CAD build for the part. Positions are in the model's coordinates, mm. Face numbers are marked on the shaded views. A direction names the side the tool comes from. Coordinates: 2 decimals unless noted, no trailing zeros. Order: outer loops, then holes, each group sorted by start corner. A loop starts at its lowest first (then second) coordinate and runs counter-clockwise, first axis right, second up. Notation, with made-up numbers: (13.5, -16.5) - (71.5, -16.5) arc R22 cw to (71.5, 10.5) - close; hole circle Ø8 at (-32.5, -33). An arc over 180 degrees is marked (long way). Write each question's results on one line, items separated by ' | '. Start each with the question number.
Q1. Which spindle directions (+Z, -Z, +X, -X, +Y, -Y) get a long thin tool onto all of the face, cutting with end or side? Do the marked faces 1 and 2. Say none if no direction does.
Q2. Wall check: probe 1 along Y at (x, z) = (-4.5, -0.75); probe 2 along X at (y, z) = (16.25, 0.5); probe 3 along X at (y, z) = (14.5, 1). Give the ranges that are in metal, low to high.
Q3. Band-saw the part on A-A, the plane y = 13.5. Write the cut outline in (x, z), then the cut area to 3 significant figures.
Q4. Pin check, flat tips, straight feed: P1, Ø1.5, axis at x = 0.5, y = 8.5, coming from the -Z side; P2, Ø2, axis at x = -3.5, y = 16.5, coming from the -Z side; P3, Ø2, axis at x = 4, z = 2, coming from the -Y side; P4, Ø3, axis at y = 13.5, z = -1, coming from the -X side. Stop position of each tip, or through.
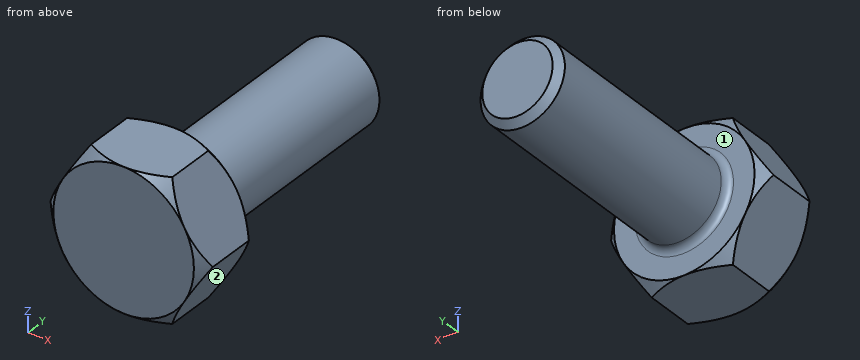
Autodesk Inventor part; units mm, degrees
ref_plane "YZ Plane" through (0, 0, 0) normal (1, 0, 0) x (0, 1, 0)
ref_plane "XZ Plane" through (0, 0, 0) normal (0, 1, 0) x (-1, 0, 0)
ref_plane "XY Plane" through (0, 0, 0) normal (0, 0, 1) x (1, 0, 0)
sketch "Esboço1" plane through (0, 0, 0) normal (0, 1, 0) x (-1, 0, 0)
  circle A0 centre (0, 0) radius 3
  line L0 (-2.8868, -5) -> (-5.7735, 0)
  line L1 (-5.7735, 0) -> (-2.8868, 5)
  line L2 (-2.8868, 5) -> (2.8868, 5)
  line L3 (2.8868, 5) -> (5.7735, 0)
  line L4 (5.7735, 0) -> (2.8868, -5)
  line L5 (2.8868, -5) -> (-2.8868, -5)
  dimension "d0" = 6
extrude "Extrusão1" add sketch "Esboço1" along normal blind 5
sketch "Esboço2" plane through (0, 0, 0) normal (1, 0, 0) x (0, 1, 0)
  point P0 (0, 0)
chamfer "Chanfro1" distance 0.5 angle 45 2 edges at (3, 0, 0) (3, 5, 0)
sketch "Esboço5" plane through (0, 0, 0) normal (0, -1, 0) x (1, 0, 0)
  circle A0 centre (0, 0) radius 5
extrude "Extrusão2" cut sketch "Esboço5" against normal through all draft 45 keep common part
sketch "Esboço6" plane through (0, 5, 0) normal (0, 1, 0) x (1, 0, 0)
  circle A0 centre (0, 0) radius 5
extrude "Extrusão3" cut sketch "Esboço6" against normal through all draft 45 keep common part
sketch "Esboço7" plane through (0, 5, 0) normal (0, 1, 0) x (1, 0, 0)
  circle A0 centre (0, 0) radius 3.5
extrude "Extrusão4" add sketch "Esboço7" against normal blind 5
sketch "Esboço8" plane through (0, 5, 0) normal (0, 1, 0) x (1, 0, 0)
  circle A0 centre (0, 0) radius 3
  dimension "d16" = 6
extrude "Extrusão5" add sketch "Esboço8" along normal blind 16
chamfer "Chanfro2" distance 0.5 angle 45 1 edges at (-3, 21, 0)
fillet "Arredondamento1" radius 0.5 1 edges at (-3, 5, 0)
thread "Rosca2"
properties part number "porca m6" material "Aço inoxidável"
Results below:
1) face 1: +Y | face 2: -Z, +X, +Y, -Y
2) probe 1: y = 0 to 5 | probe 2: x = -2.96 to 2.96 | probe 3: x = -2.83 to 2.83
3) outline: circle Ø6 at (0, 0) | area: 28.3 mm²
4) P1: stops at z = -3 | P2: stops at z = -1.66 | P3: stops at y = 0 | P4: stops at x = -3
